Source: CAD feature listing. Evaluate the final solid. Frame: model axes, mm. Round coordinates to 2 decimals unless told otherwise and drop trailing zeros. Loops run counter-clockwise (first coordinate to the right, second up) from the corner with the lowest first, then second, coordinate; pieces in that order, holes last.
(1) Material intervals for probe 1 along Y at (x, z) = (200, 2); probe 2 along Y at (x, z) = (390, 1.6); probe 3 along Y at (x, z) = (300, 2.2), sorted ascending.
(2) First-contact query: pin 1 Ø22.5 at (x, y) = (300, 79.64) entering from -Z. Flat tip, straight axial feed; report the tip coordinate or a pass-through.
(3) Section B-B, the plane y = 24.5. Count the separate pieces of the cut face and the enclosed holes in it, plus the area to 3 significant figures.
(4) Section D-D, the plane y = 56.5. Return the cut outline in (x, z).
(5) Section A-A, the plane x = 250. Return the cut outline in (y, z), plus the area to 3 significant figures.
```python
from build123d import *

# Parameters (mm, degrees)
SKETCH1_W           = 400
SKETCH1_H           = 100
SKETCH1_R           = 35
SKETCH1_R_2         = 12.5
SKETCH1_R_3         = 2.5
BOSS_EXTRUDE1_DEPTH = 4
FILLET1_R           = 10


with BuildPart() as part:
    # Sketch1 → Boss-Extrude1 (new body)
    with BuildSketch(Plane.XY):
        with Locations((200, 50)):
            Rectangle(SKETCH1_W, SKETCH1_H)
        with Locations((50, 50)):
            Circle(SKETCH1_R, mode=Mode.SUBTRACT)
        with Locations((150, 50)):
            Circle(SKETCH1_R, mode=Mode.SUBTRACT)
        with Locations((250, 50)):
            Circle(SKETCH1_R, mode=Mode.SUBTRACT)
        with Locations((350, 50)):
            Circle(SKETCH1_R, mode=Mode.SUBTRACT)
        with Locations((100, 79.642297689)):
            Circle(SKETCH1_R_2, mode=Mode.SUBTRACT)
        with Locations(Location((100, 20.357702311, 0), (0, 0, 180))):
            Circle(SKETCH1_R_2, mode=Mode.SUBTRACT)
        with Locations(Location((200, 20.357702311, 0), (0, 0, 180))):
            Circle(SKETCH1_R_2, mode=Mode.SUBTRACT)
        with Locations((200, 79.642297689)):
            Circle(SKETCH1_R_2, mode=Mode.SUBTRACT)
        with Locations(Location((300, 20.357702311, 0), (0, 0, 180))):
            Circle(SKETCH1_R_2, mode=Mode.SUBTRACT)
        with Locations((300, 79.642297689)):
            Circle(SKETCH1_R_2, mode=Mode.SUBTRACT)
        with Locations((10, 10)):
            Circle(SKETCH1_R_3, mode=Mode.SUBTRACT)
        with Locations(Location((10, 90, 0), (0, 0, 180))):
            Circle(SKETCH1_R_3, mode=Mode.SUBTRACT)
        with Locations((390, 90)):
            Circle(SKETCH1_R_3, mode=Mode.SUBTRACT)
        with Locations(Location((390, 10, 0), (0, 0, 180))):
            Circle(SKETCH1_R_3, mode=Mode.SUBTRACT)
        with Locations((200, 50)):
            Circle(SKETCH1_R_3, mode=Mode.SUBTRACT)
    extrude(amount=BOSS_EXTRUDE1_DEPTH)

    # Fillet1
    fillet1_edges = [part.edges().sort_by_distance(p)[0] for p in [
        (0, 100, 2),
        (400, 100, 2),
        (400, 0, 2),
        (0, 0, 2),
    ]]
    fillet(fillet1_edges, radius=FILLET1_R)


solid = part.part
```
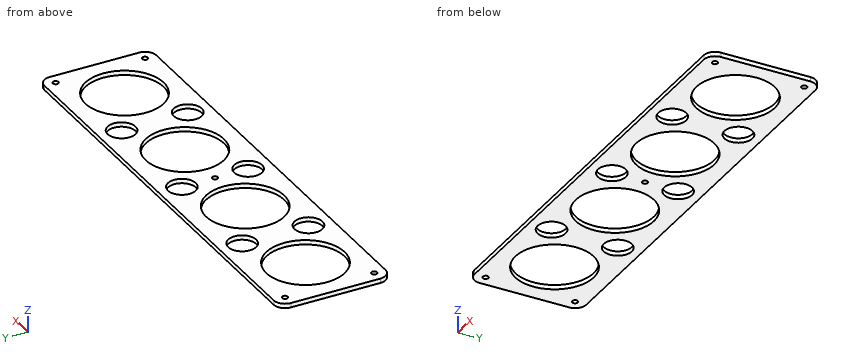
Output values:
1. probe 1: y = 0 to 7.86, 32.86 to 47.5, 52.5 to 67.14, 92.14 to 100
1. probe 2: y = 0 to 7.5, 12.5 to 87.5, 92.5 to 100
1. probe 3: y = 0 to 7.86, 32.86 to 67.14, 92.14 to 100
2. pin 1: passes through
3. separate pieces: 8
3. enclosed holes: 0
3. area: 550 mm2
4. outline: (0, 0) - (15.61, 0) - (15.61, 4) - (0, 4) - close; (84.39, 0) - (115.61, 0) - (115.61, 4) - (84.39, 4) - close; (184.39, 0) - (215.61, 0) - (215.61, 4) - (184.39, 4) - close; (284.39, 0) - (315.61, 0) - (315.61, 4) - (284.39, 4) - close; (384.39, 0) - (400, 0) - (400, 4) - (384.39, 4) - close
5. outline: (0, 0) - (15, 0) - (15, 4) - (0, 4) - close; (85, 0) - (100, 0) - (100, 4) - (85, 4) - close
5. area: 120 mm2
